The listing builds one solid part. Answer for the finished solid, in the listing's coordinates (mm). Give positions to 0.01 mm unless a question says otherwise; leave off trailing zeros. Loops run counter-clockwise (first coordinate to the right, second up) from the corner with the lowest first, then second, coordinate; pieces in that order, holes last. Notation, with made-up numbers: M 10.5,81.5 L 30.5,81.5 A28 ccw 30.5,108.5 Z; hole C -36.75,-26 d10. An arc over 180 degrees is marked long. Return JSON: item names as keys, results as strings.
Autodesk Inventor part; units mm, degrees
ref_plane "YZ Plane" through (0, 0, 0) normal (1, 0, 0) x (0, 1, 0)
ref_plane "XZ Plane" through (0, 0, 0) normal (0, 1, 0) x (-1, 0, 0)
ref_plane "XY Plane" through (0, 0, 0) normal (0, 0, 1) x (1, 0, 0)
sketch "Sketch1" plane through (0, 0, 0) normal (1, 0, 0) x (0, 1, 0)
  line L0 (0, 0) -> (10, 0)
  line L1 (10, 0) -> (10, -200)
  line L2 (10, -200) -> (0, -200)
  line L3 (0, -200) -> (0, 0)
  dimension "d0" = 10
  dimension "d1" = 200
extrude "Extrusion1" add sketch "Sketch1" along normal blind 3
sketch "Sketch2" plane through (3, 0, 0) normal (1, 0, 0) x (0, 0, -1)
  line L0 (0, 10) -> (0, 0)
  line L1 (0, 0) -> (200, 0)
  line L2 (0, 10) -> (10, 10)
  line L3 (10, 10) -> (10, 0)
  line L4 (10, 0) -> (0, 0)
  line L5 (0, 0) -> (0, 10)
  line L6 (200, 0) -> (200, 10)
  line L7 (200, 10) -> (190, 10)
  line L8 (190, 10) -> (190, 0)
  line L9 (190, 0) -> (200, 0)
  line L10 (200, 0) -> (200, 10)
  dimension "d4" = 10
  dimension "d5" = 10
extrude "Extrusion2" add sketch "Sketch2" along normal blind 60
sketch "Sketch3" plane through (63, 0, 0) normal (1, 0, 0) x (0, 0, -1)
  line L0 (0, 10) -> (200, 10) construction
  line L1 (10, 0) -> (190, 0) construction
  line L2 (0, 10) -> (10, 0) construction
  line L3 (5, 5) -> (0, 5) construction
  line L4 (0, 0) -> (0, 10) construction
  circle A0 centre (5, 5) radius 3.175
  line L5 (200, 10) -> (190, 10) construction
  line L6 (200, 0) -> (200, 10) construction
  line L7 (190, 10) -> (200, 0) construction
  circle A1 centre (195, 5) radius 3.175
  dimension "d8" = 6.35
  dimension "d9" = 6.35
extrude "Extrusion3" cut sketch "Sketch3" against normal blind 30
sketch "Sketch4" plane through (0, 0, -200) normal (0, 0, -1) x (-1, 0, 0)
  line L0 (0, 0) -> (-63, 0) construction
  line L1 (0, 0) -> (-20, 0) construction
  line L2 (-20, 0) -> (-20, 20) construction
  line L3 (-20, 20) -> (0, 20) construction
  line L4 (0, 20) -> (0, 0) construction
  line L5 (-3, 10) -> (-63, 10) construction
  circle A0 centre (-10, 10) radius 8 construction
  line L6 (0, 10) -> (-63, 10)
  arc A1 (-2, 10) -> (-18, 10) centre (-10, 10) ccw
  line L7 (-20, 10) -> (-18, 10)
  line L8 (-2, 10) -> (0, 10)
  line L9 (0, 20) -> (-20, 20)
  line L10 (-20, 10) -> (-20, 20)
  line L11 (0, 20) -> (0, 10)
  dimension "d12" = 20
  dimension "d13" = 20
  dimension "d14" = 16
extrude "Extrusion4" add sketch "Sketch4" against normal blind 10 contours L6 A1 L10 L9 L11
fillet "Fillet1" radius 5 2 edges at (0, 20, -195) (20, 20, -195)
fillet "Fillet2" radius 5 1 edges at (20, 10, -195)
sketch "Sketch5" plane through (63, 0, -200) normal (0, 0, -1) x (-1, 0, 0)
  arc A0 (61, 10) -> (45, 10) centre (53, 10) ccw
  circle A1 centre (53, 10) radius 8
  point P0 (63, 0)
extrude "Extrusion5" cut sketch "Sketch5" against normal blind 200
sketch "Sketch6" plane through (3, 0, -190) normal (0, 0, 1) x (1, 0, 0)
  arc A0 (0, 6.127) -> (-1, 10) centre (7, 10) ccw
  circle A1 centre (7, 10) radius 8
  circle A2 centre (7, 10) radius 5
  point P0 (-3, 0)
  dimension "d21" = 10
extrude "Extrusion6" add sketch "Sketch6" against normal blind 5
sketch "Sketch7" plane through (0, 0, 0) normal (0, 0, 1) x (1, 0, 0)
  line L0 (0, 0) -> (63, 0) construction
  line L1 (0, 0) -> (20, 0) construction
  line L2 (20, 0) -> (20, 20) construction
  line L3 (20, 20) -> (0, 20) construction
  line L4 (0, 20) -> (0, 0) construction
  circle A0 centre (10, 10) radius 8 construction
  line L5 (2, 10) -> (0, 10)
  line L6 (2, 10) -> (0, 10)
  line L7 (0, 10) -> (0, 20)
  line L8 (20, 20) -> (0, 20)
  line L9 (20, 20) -> (20, 10)
  line L10 (18, 10) -> (63, 10)
  line L11 (18, 10) -> (20, 10)
  arc A1 (18, 10) -> (2, 10) centre (10, 10) ccw
  dimension "d24" = 20
  dimension "d25" = 20
  dimension "d26" = 16
extrude "Extrusion7" add sketch "Sketch7" against normal blind 10
fillet "Fillet3" radius 5 3 edges at (0, 20, -5) (20, 20, -5) (20, 10, -5)
sketch "Sketch8" plane through (63, 0, -10) normal (0, 0, -1) x (-1, 0, 0)
  circle A0 centre (53, 10) radius 5
  circle A1 centre (53, 10) radius 5
  circle A2 centre (53, 10) radius 8
  point P0 (63, 0)
extrude "Extrusion8" add sketch "Sketch8" against normal blind 5
sketch "Sketch9" plane through (63, 0, -10) normal (0, 0, -1) x (-1, 0, 0)
  line L0 (63, 0) -> (43, 0)
  line L1 (43, 0) -> (43, 2)
  line L2 (43, 2) -> (63, 2)
  line L3 (63, 2) -> (63, 0)
  dimension "d32" = 20
  dimension "d33" = 2
extrude "Extrusion9" add sketch "Sketch9" along normal blind 190
sketch "Sketch10" plane through (3, 2, -10) normal (0, 1, 0) x (1, 0, 0)
  line L0 (17, 180) -> (14, 180)
  line L1 (14, 180) -> (14, 0)
  line L2 (14, 0) -> (17, 0)
  line L3 (17, 0) -> (17, 180)
  point P0 (-3, -10)
  dimension "d36" = 3
sketch "Sketch11" plane through (0, 10, -10) normal (0, 1, 0) x (1, 0, 0)
  line L0 (3, 180) -> (3, 0)
  line L1 (0, 180.0445) -> (3, 180.0445)
  line L2 (3, 180.0445) -> (3, 0)
  line L3 (3, 0) -> (0, 0)
  line L4 (0, 0) -> (0, 180.0445)
  point P0 (0, -10)
extrude "Extrusion10" add sketch "Sketch11" against normal blind 10
extrude "Extrusion11" add sketch "Sketch10" along normal blind 6
properties part number "rearAxelHolder 6-5"
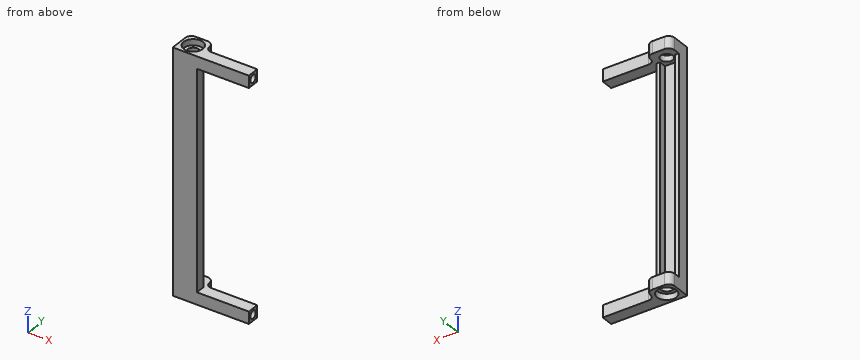
(1) The part is cut by section A-A (x = 44). Determine the outline of the cut face in (y, z) (3 decimals).
Values follow:
{"outline": "M 0,-200 L 10,-200 L 10,-190 L 0,-190 Z; M 0,-10 L 10,-10 L 10,0 L 0,0 Z; hole C 5,-195 d6.35; hole C 5,-5 d6.35"}
(2) Straight lines are drawn through the part: line 1 along X through (y, z) = (7.5, -121.5); line 2 along Y through (x, z) = (40.75, -5) (3 decimals); line 3 along Z through (x, y) = (22, 10.75). For each, find the intervals that lie inside material, in ascending order.
Values follow:
{"line 1": "0 to 3, 17 to 20", "line 2": "0 to 1.825, 8.175 to 10", "line 3": "-200 to -190, -10 to 0"}
(3) Given pin 1 (3.5 mm diameter, centred on x = 1, z = -93.5, fed in from +Y); pin 2 (5 mm diameter, centred on x = 6.5, y = 10, fed in from -Z); pin 3 (2.5 mm diameter, centred on y = 5, z = -107, fed in from +X), each flat-ended and moving along its own axis, determine where each tip first touches the part or whether it passes through.
Values follow:
{"pin 1": "y = 10", "pin 2": "z = -195", "pin 3": "x = 20"}
(4) The part is cut by section D-D (y = 12). Determine the outline of the cut face in (x, z), and give its area (3 significant figures).
Values follow:
{"outline": "M 0,-200 L 2.25,-200 L 2.25,-195 L 5.42,-195 L 5.42,-190 L 0,-190 Z; M 0,-10 L 5.42,-10 L 5.42,-5 L 2.25,-5 L 2.25,0 L 0,0 Z; M 14.58,-195 L 17.75,-195 L 17.75,-200 L 21,-200 L 21,-190 L 14.58,-190 Z; M 14.58,-10 L 21,-10 L 21,0 L 17.75,0 L 17.75,-5 L 14.58,-5 Z", "area": "173 mm²"}
(5) The part is cut by section C-C (z = -106). Determine the outline of the cut face in (x, y).
Values follow:
{"outline": "M 0,0 L 20,0 L 20,8 L 17,8 L 17,2 L 3,2 L 3,10 L 0,10 Z"}
(6) The part is cut by section B-B (x = 10). Determine the outline of the cut face in (y, z), and give its area (3 significant figures).
Values follow:
{"outline": "M 0,-200 L 2,-200 L 2,-195 L 5,-195 L 5,-190 L 2,-190 L 2,-10 L 5,-10 L 5,-5 L 2,-5 L 2,0 L 0,0 Z; M 15,-195 L 18,-195 L 18,-200 L 20,-200 L 20,-190 L 15,-190 Z; M 15,-10 L 20,-10 L 20,0 L 18,0 L 18,-5 L 15,-5 Z", "area": "500 mm²"}
